Geometry check sheet. Reference: the model listing, model coordinates, mm. Coordinates: 2 decimals unless noted, no trailing zeros. Write each loop counter-clockwise with the first axis right and the second up, starting at its lowest first coordinate (ties: lowest second). Pieces come first, ordered by that corner, then holes. Notation, with made-up numbers: M 63,-4.75 L 92,-4.75 A13 ccw 92,18.25 Z; hole C 66.25,10 d11. An arc over 180 degrees is marked long. Write each question's results on one line, items separated by ' | '.
```python
from build123d import *

# Parameters (mm, degrees)
ESQUISSE1_W             = 15
ESQUISSE1_H             = 60
BOSS_EXTRU_1_DEPTH      = 15
ESQUISSE2_W             = 10
ESQUISSE2_H             = 8.70960714
ESQUISSE2_H_2           = 11.830290252
ENL_V_MAT_EXTRU_1_DEPTH = 183.619823677
ESQUISSE3_W             = 15
ESQUISSE3_H             = 15
ESQUISSE3_W_2           = 45
BOSS_EXTRU_2_DEPTH      = 15


with BuildPart() as part:
    # Esquisse1 → Boss.-Extru.1 (new body)
    with BuildSketch(Plane.XY):
        with BuildLine():
            ThreePointArc((-175, -30), (-169.142135624, -44.142135624), (-155, -50))
            Line((-155, -50), (155, -50))
            ThreePointArc((155, -50), (169.142135624, -44.142135624), (175, -30))
            Line((175, -30), (175, 30))
            ThreePointArc((175, 30), (169.142135624, 44.142135624), (155, 50))
            Line((155, 50), (-155, 50))
            ThreePointArc((-155, 50), (-169.142135624, 44.142135624), (-175, 30))
            Line((-175, 30), (-175, -30))
        make_face()
        with Locations((-147.5, 0)):
            Rectangle(ESQUISSE1_W, ESQUISSE1_H, mode=Mode.SUBTRACT)
        Polygon((-52.61, -30), (-60.11, -30), (-60.11, -20), (-52.61, -20), (-52.61, -4.714066344), (-42.61, -4.714066344), (-42.61, -20), (-35.11, -20), (-35.11, -30), (-42.61, -30), (-42.61, -45.27278392), (-52.61, -45.27278392), align=None, mode=Mode.SUBTRACT)
        Polygon((42.61, -30), (35.11, -30), (35.11, -20), (42.61, -20), (42.61, -4.714066344), (52.61, -4.714066344), (52.61, -20), (60.11, -20), (60.11, -30), (52.61, -30), (52.61, -45.27278392), (42.61, -45.27278392), align=None, mode=Mode.SUBTRACT)
        with Locations((-102.5, 0)):
            Rectangle(ESQUISSE1_W, ESQUISSE1_H, mode=Mode.SUBTRACT)
        with Locations((102.5, 0)):
            Rectangle(ESQUISSE1_W, ESQUISSE1_H, mode=Mode.SUBTRACT)
        with Locations((147.5, 0)):
            Rectangle(ESQUISSE1_W, ESQUISSE1_H, mode=Mode.SUBTRACT)
    extrude(amount=BOSS_EXTRU_1_DEPTH)

    # Esquisse2 → Enlèv. mat.-Extru.1 (cut, through all)
    with BuildSketch(Plane.XY.offset(15)):
        with Locations((47.61, -49.62758749)):
            Rectangle(ESQUISSE2_W, ESQUISSE2_H)
        with Locations((-47.61, -51.187929046)):
            Rectangle(ESQUISSE2_W, ESQUISSE2_H_2)
    extrude(amount=-ENL_V_MAT_EXTRU_1_DEPTH, mode=Mode.SUBTRACT)

    # Esquisse3 → Boss.-Extru.2 (add)
    with BuildSketch(Plane(origin=(0, -50, 0), x_dir=(-1, 0, 0), z_dir=(0, -1, 0))):
        with Locations((-70.11, -7.5)):
            Rectangle(ESQUISSE3_W, ESQUISSE3_H)
        with Locations((10.11, -7.5)):
            Rectangle(ESQUISSE3_W_2, ESQUISSE3_H)
        with Locations((70.11, -7.5)):
            Rectangle(ESQUISSE3_W, ESQUISSE3_H)
    extrude(amount=BOSS_EXTRU_2_DEPTH)


solid = part.part
```
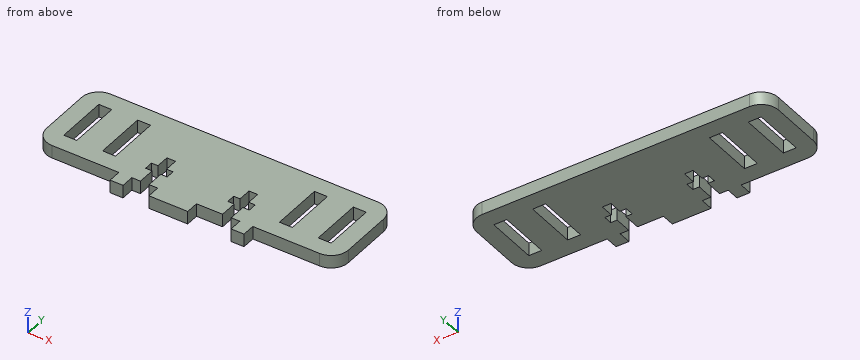
Q1. Sectioned sample at B-B on y = -54. Record the cut outline in (x, z), and give its area (4 significant figures).
Geometry check:
outline: M -77.61,0 L -62.61,0 L -62.61,15 L -77.61,15 Z; M -32.61,0 L 12.39,0 L 12.39,15 L -32.61,15 Z; M 62.61,0 L 77.61,0 L 77.61,15 L 62.61,15 Z | area: 1,125 mm2
Q2. Sectioned sample at A-A on y = 20. Record the cut outline in (x, z), and give its area (3 significant figures).
Geometry check:
outline: M -175,0 L -155,0 L -155,15 L -175,15 Z; M -140,0 L -110,0 L -110,15 L -140,15 Z; M -95,0 L 95,0 L 95,15 L -95,15 Z; M 110,0 L 140,0 L 140,15 L 110,15 Z; M 155,0 L 175,0 L 175,15 L 155,15 Z | area: 4,350 mm2
Q3. Depth check by flat-ended pin: P1, Ø7.5, axis at y = -57.5, z = 5, coming from the -X side; P2, Ø7.5, axis at y = -60, z = 7, coming from the +X side; P3, Ø2, axis at x = 37, z = 4, coming from the -Y side. Enter the tip coordinate at first touch or a pass-through.
Geometry check:
P1: stops at x = -77.61 | P2: stops at x = 77.61 | P3: stops at y = -50
Q4. Scan lines: probe 1 along X at (y, z) = (-1.5, 6); probe 2 along X at (y, z) = (-50.5, 11.75); probe 3 along Y at (x, z) = (-60, 8.75). Record each from-to range of solid material in increasing order.
Geometry check:
probe 1: x = -175 to -155, -140 to -110, -95 to 95, 110 to 140, 155 to 175 | probe 2: x = -77.61 to -62.61, -32.61 to 12.39, 62.61 to 77.61 | probe 3: y = -50 to -30, -20 to 50
Q5. Sectioned sample at C-C on z = 2.5. Give the number of separate pieces and of enclosed holes in the cut face, and give its area (3 significant figures).
Geometry check:
separate pieces: 1 | enclosed holes: 4 | area: 31,000 mm2
